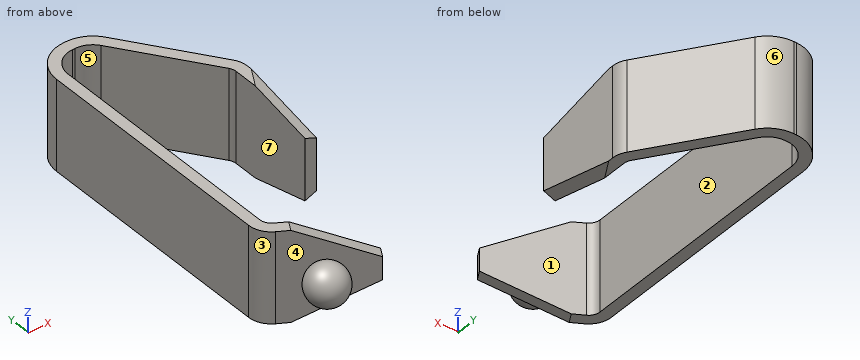
```python
from build123d import *

# Parameters (mm, degrees)
EXTRUDE_THIN1_DEPTH     = 2
CUT_EXTRUDE1_DEPTH      = 14.670442165
CUT_EXTRUDE1_DEPTH_BACK = 14.670442165


with BuildPart() as part:
    # Sketch1 → Extrude-Thin1 (new, symmetric)
    with BuildSketch(Plane.XY):
        with BuildLine():
            Line((3.5, -2.020725942), (0.25, -0.144337567))
            ThreePointArc((0.25, -0.144337567), (0.066987298, 0.038675135), (0, 0.288675135))
            Line((0, 0.288675135), (0, 11))
            ThreePointArc((0, 11), (0.292893219, 11.707106781), (1, 12))
            Line((1, 12), (1.1, 12))
            ThreePointArc((1.1, 12), (1.561748613, 11.887010833), (1.919152044, 11.573576436))
            Line((1.919152044, 11.573576436), (4.570098185, 7.787632989))
            ThreePointArc((4.570098185, 7.787632989), (4.637380639, 7.651197671), (4.660522163, 7.500844771))
            Line((4.660522163, 7.500844771), (4.660522163, 3.658494165))
            Line((4.660522163, 3.658494165), (5.160522163, 3.658494165))
            Line((5.160522163, 3.658494165), (5.160522163, 7.500844771))
            ThreePointArc((5.160522163, 7.500844771), (5.114239114, 7.80155057), (4.979674208, 8.074421207))
            Line((4.979674208, 8.074421207), (2.328728066, 11.860364655))
            ThreePointArc((2.328728066, 11.860364655), (1.79262292, 12.33051625), (1.1, 12.5))
            Line((1.1, 12.5), (1, 12.5))
            ThreePointArc((1, 12.5), (-0.060660172, 12.060660172), (-0.5, 11))
            Line((-0.5, 11), (-0.5, 0.288675135))
            ThreePointArc((-0.5, 0.288675135), (-0.366025404, -0.211324865), (0, -0.577350269))
            Line((0, -0.577350269), (3.25, -2.453738644))
            Line((3.25, -2.453738644), (3.5, -2.020725942))
        make_face()
    extrude(amount=EXTRUDE_THIN1_DEPTH, both=True)

    # Sketch3 → Cut-Extrude1 (cut, two sides: drawn at the far end of the back side and taken through both)
    with BuildSketch(Plane(origin=(0, 0, 0), x_dir=(0.8660254037844364, -0.500000000000004, 0), z_dir=(0.500000000000004, 0.8660254037844364, 0)).offset(-CUT_EXTRUDE1_DEPTH_BACK)):
        Polygon((33.065052182, 13.033927086), (4.041451884, -0.5), (0.824691504, -2), (0.824691504, -2.582001287), (5.059767422, -2.582001287), (5.059767422, 2.96154049), (0.824691504, 2.96154049), (0.824691504, 2), (4.041451884, 0.5), (33.065052182, -13.033927086), (97.113051575, -13.033927086), (97.113051575, 13.033927086), align=None)
    extrude(amount=CUT_EXTRUDE1_DEPTH + CUT_EXTRUDE1_DEPTH_BACK, mode=Mode.SUBTRACT)

    # Sketch6 → Revolve1 (revolve)
    with BuildSketch(Plane.XY):
        with BuildLine():
            Line((1.482050808, -1.433012702), (2.00166605, -1.733012702))
            ThreePointArc((2.00166605, -1.733012702), (1.705049292, -2.662317438), (0.732050808, -2.732050808))
            Line((0.732050808, -2.732050808), (1.482050808, -1.433012702))
        make_face()
    revolve(axis=Axis((1.482050808, -1.433012702, 0), (-0.5000000000000001, -0.8660254037844387, 0)))


solid = part.part
```
Can you work these out from the model? Positions are in its coordinate system, mm. Face numbers are marked on the shaded views. A direction names the side the tool comes from. Give positions to 0.01 mm unless a question says otherwise; leave off trailing zeros. Order: outer loops, then holes, each group sorted by start corner. A loop starts at its lowest first (then second) coordinate and runs counter-clockwise, first axis right, second up. Notation, with made-up numbers: (43.5, 36.5) - (90.5, 36.5) arc R16 cw to (90.5, 57.5) - close; hole circle Ø4 at (41.25, 78.5). An arc over 180 degrees is marked (long way). Use a Markdown table: item, result. Add a question column.
Q1. If we section it at D-D on x = 2.8: Write out the boundary of the cut face in (y, z), plus the area to 3 significant figures.
Q2. If we section it at A-A on x = 1.75: Write out the boundary of the cut face in (y, z), plus the area to 3 significant figures.
Q3. I'm going to push flat-ended pins straight in: pin 1 (1.5 mm diameter, centred on x = 2, y = 10, fed in from +Z); pin 2 (2 mm diameter, centred on y = 1, z = -1.5, fed in from +X). Where does each tip first touch, or does it pass through?
Q4. If we section it at C-C on z = 0.35: Write out the boundary of the cut face in (x, y).
Q5. If we section it at B-B on y = 5: Write out the boundary of the cut face in (x, z), plus the area to 3 significant figures.
Q6. On a 3-axis mill with a long thin cutter (end or side, diameter ignored), from which of +Z, -Z, +X, -X, +Y, -Y can I reach the whole of each face in a straight line? I mean the marked faces 5, 6 and 7. Say none if no direction works.
Q7. Please list where these lines run through material, in increasing order: line 1 along X through (y, z) = (5.5, -1.5); line 2 along X through (y, z) = (0.5, 0.2); line 3 along Y through (x, z) = (0.6, 0.5).
Q8. If we mould it in two halves opening along X, with no side actions, what happens to the marked faces 1, 2, 3 and 4? For each: released by +X, released by -X, zero draft, split by the parting line, or undercut.
Answers follow:
| question | item | result |
|---|---|---|
| 1 | outline | (-2.19, -0.74) - (-1.62, -0.88) - (-1.62, 0.88) - (-2.19, 0.74) - close; (10.32, -2) - (11.19, -2) - (11.19, 2) - (10.32, 2) - close |
| 1 | area | 4.42 mm^2 |
| 2 | outline | (-1.59, -1.31) - (-1.01, -1.44) - (-1.01, 1.44) - (-1.59, 1.31) - (-1.59, 0.51) arc R0.65 ccw (long way) to (-1.59, -0.51) - close; (11.76, -2) - (12.35, -2) - (12.35, 2) - (11.76, 2) - close |
| 2 | area | 5.08 mm^2 |
| 3 | pin 1 | passes through |
| 3 | pin 2 | stops at x = 0.09 |
| 4 | outline | (-0.5, 0.29) arc R1 ccw to (0, -0.58) - (1.06, -1.19) arc R0.8 ccw (long way) to (1.9, -1.68) - (3.25, -2.45) - (3.5, -2.02) - (0.25, -0.14) arc R0.5 cw to (0, 0.29) - (0, 11) arc R1 cw to (1, 12) - (1.1, 12) arc R1 cw to (1.92, 11.57) - (4.57, 7.79) arc R0.5 cw to (4.66, 7.5) - (4.66, 3.66) - (5.16, 3.66) - (5.16, 7.5) arc R1 ccw to (4.98, 8.07) - (2.33, 11.86) arc R1.5 ccw to (1.1, 12.5) - (1, 12.5) arc R1.5 ccw to (-0.5, 11) - close |
| 5 | outline | (-0.5, -2) - (0, -2) - (0, 2) - (-0.5, 2) - close; (4.66, -1.67) - (5.16, -1.47) - (5.16, 1.47) - (4.66, 1.67) - close |
| 5 | area | 3.57 mm^2 |
| 6 | face 5 | +Z, -Z |
| 6 | face 6 | +Z, -Z, +X, +Y |
| 6 | face 7 | +Z, -Z, -Y |
| 7 | line 1 | x = -0.5 to 0, 4.66 to 5.16 |
| 7 | line 2 | x = -0.5 to 0 |
| 7 | line 3 | y = -2.41 to -1.55, -0.92 to -0.35, 11.92 to 12.45 |
| 8 | face 1 | released by +X |
| 8 | face 2 | undercut |
| 8 | face 3 | released by -X |
| 8 | face 4 | undercut |
